Geometry check sheet. Reference: the model listing, model coordinates, mm. Face numbers are marked on the shaded views. A direction names the side the tool comes from. Give positions to 0.01 mm unless a question says otherwise; leave off trailing zeros. Loops run counter-clockwise (first coordinate to the right, second up) from the corner with the lowest first, then second, coordinate; pieces in that order, holes last. Notation, with made-up numbers: (-30.5, 54.5) -> (17.5, 54.5) arc R34 cw to (17.5, 86.5) -> close; hole circle Ø9 at (56, 51.25). An arc over 180 degrees is marked (long way). One line per item, written item: value. Start each with the question number.
(1) Sectioned sample at D-D, the plane z = 5. Record the cut outline in (x, y).
(2) Sectioned sample at A-A, the plane z = -5. Record the cut outline in (x, y) (3 decimals), then the cut area to 3 significant figures.
(3) Scan lines: line 1 along X through (y, z) = (-2.25, 3); line 2 along Z through (x, y) = (-3.25, 1); line 3 along X through (y, z) = (0, -2). Record each from-to range of solid material in increasing order. Write a range as from..to.
(4) Tool access check on the marked faces 4 and 5. Record the directions out of +Z, -Z, +X, -X, +Y, -Y that give a thin tool (end or side, any length) a straight path to the whole face; none if there is none.
(5) Draft check along Z on the marked faces 1, 2 and 3. Enter one of: pulls with the +Z half, pulls with the -Z half, needs draft (parallel to the pull), parting line crosses it, or undercut.
(6) Gauge pin test, flat ends, axial feed: pin 1 Ø6 at (x, z) = (-13, 2.5) entering from +Y (3 decimals); pin 2 Ø1.5 at (y, z) = (3, -19.5) entering from +X; pin 3 Ø5 at (y, z) = (1, -21) entering from -X; pin 4 Ø3.5 at (x, z) = (-4.88, 10.87) entering from -Y. Record the tip position at first contact, or that the pin passes through.
(7) Sectioned sample at C-C, the plane y = 4. Record the cut outline in (x, z).
(8) Sectioned sample at B-B, the plane x = 4.5. Record the cut outline in (y, z), then the cut area to 3 significant figures.
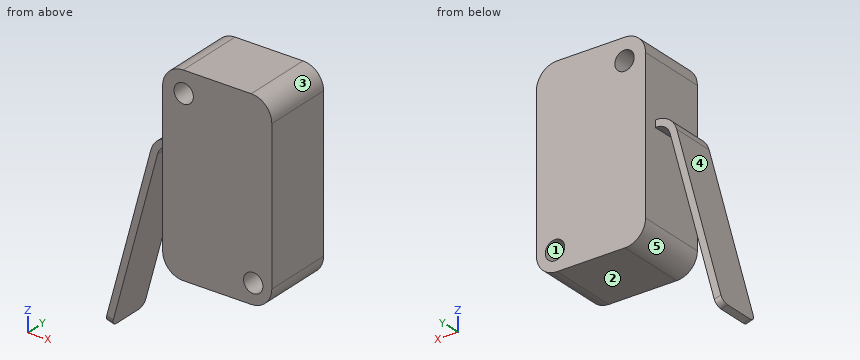
from build123d import *

# Parameters (mm, degrees)
SKETCH1_W           = 15.9004
SKETCH1_H           = 27.94
BOSS_EXTRUDE1_DEPTH = 5.08
FILLET1_R           = 3
BOSS_EXTRUDE2_DEPTH = 3.175
FILLET2_R           = 1
SKETCH3_R           = 1.4097
CUT_EXTRUDE1_DEPTH  = 16.35


with BuildPart() as part:
    # Sketch1 → Boss-Extrude1 (new, symmetric)
    with BuildSketch(Plane(origin=(0, 0, 0), x_dir=(1, 0, 0), z_dir=(0, 1, 0))):
        Rectangle(SKETCH1_W, SKETCH1_H)
    extrude(amount=BOSS_EXTRUDE1_DEPTH, both=True)

    # Fillet1
    fillet1_edges = [part.edges().sort_by_distance(p)[0] for p in [
        (7.9502, 0, 13.97),
        (-7.9502, 0, 13.97),
        (-7.9502, 0, -13.97),
        (7.9502, 0, -13.97),
    ]]
    fillet(fillet1_edges, radius=FILLET1_R)

    # Sketch2 → Boss-Extrude2 (add, symmetric)
    with BuildSketch(Plane(origin=(0, 0, 0), x_dir=(1, 0, 0), z_dir=(0, 1, 0))):
        with BuildLine():
            Line((-17.773175009, 24.379180955), (-11.074445198, -0.620819045))
            ThreePointArc((-11.074445198, -0.620819045), (-10.002952006, -2.224421931), (-8.176667719, -2.84436191))
            Line((-8.176667719, -2.84436191), (-3.749367894, -2.84436191))
            Line((-3.749367894, -2.84436191), (-3.749367894, -1.84436191))
            Line((-3.749367894, -1.84436191), (-8.176667719, -1.84436191))
            ThreePointArc((-8.176667719, -1.84436191), (-9.394190577, -1.43106859), (-10.108519372, -0.362))
            Line((-10.108519372, -0.362), (-16.807249182, 24.638))
            Line((-16.807249182, 24.638), (-17.773175009, 24.379180955))
        make_face()
    extrude(amount=BOSS_EXTRUDE2_DEPTH, both=True)

    # Fillet2
    fillet2_edges = [part.edges().sort_by_distance(p)[0] for p in [
        (-17.290212095, 3.175, -24.508590477),
        (-17.290212095, -3.175, -24.508590477),
    ]]
    fillet(fillet2_edges, radius=FILLET2_R)

    # Sketch3 → Cut-Extrude1 (cut)
    with BuildSketch(Plane(origin=(0, 5.08, 0), x_dir=(1, 0, 0), z_dir=(0, 1, 0))):
        with Locations(Location((5.248249785, 11.033336761, 0), (0, 0, 270))):
            Circle(SKETCH3_R)
        with Locations(Location((-4.884430829, -10.866108062, 0), (0, 0, 270))):
            Circle(SKETCH3_R)
    extrude(amount=-CUT_EXTRUDE1_DEPTH, mode=Mode.SUBTRACT)


solid = part.part
Calculated:
1. outline: (-7.95, -5.08) -> (7.95, -5.08) -> (7.95, 5.08) -> (-7.95, 5.08) -> close
2. outline: (-12.581, -3.175) -> (-11.545, -3.175) -> (-11.545, 3.175) -> (-12.581, 3.175) -> close; (-7.95, -5.08) -> (7.95, -5.08) -> (7.95, 5.08) -> (-7.95, 5.08) -> close
2. area: 168 mm2
3. line 1: x = -7.95..7.95
3. line 2: z = -13.97..13.97
3. line 3: x = -11.78..-10.74, -7.95..7.95
4. face 4: +Z, -X, +Y, -Y
4. face 5: -Z, +Y, -Y
5. face 1: undercut
5. face 2: pulls with the -Z half
5. face 3: pulls with the +Z half
6. pin 1: stops at y = 3.175
6. pin 2: stops at x = -15.23
6. pin 3: stops at x = -17.54
6. pin 4: stops at y = -5.08
7. outline: (-7.95, -10.97) arc R3 ccw to (-4.95, -13.97) -> (4.95, -13.97) arc R3 ccw to (7.95, -10.97) -> (7.95, 10.97) arc R3 ccw to (4.95, 13.97) -> (-4.95, 13.97) arc R3 ccw to (-7.95, 10.97) -> close; hole circle Ø2.82 at (-4.88, 10.87); hole circle Ø2.82 at (5.25, -11.03)
8. outline: (-5.08, -13.97) -> (5.08, -13.97) -> (5.08, -12.23) -> (-5.08, -12.23) -> close; (-5.08, -9.84) -> (5.08, -9.84) -> (5.08, 13.97) -> (-5.08, 13.97) -> close
8. area: 260 mm2
